from build123d import *

# Parameters (mm, degrees)
F0_R     = 2
F1_DEPTH = 3.2


with BuildPart() as f1:
    # F0 (on Top) → F1 (new body)
    with BuildSketch(Plane.XY):
        with BuildLine():
            ThreePointArc((0, 4), (1.171573, 1.171573), (4, 0))
            Line((4, 0), (76, 0))
            ThreePointArc((76, 0), (78.828427, 1.171573), (80, 4))
            Line((80, 4), (80, 86.6))
            ThreePointArc((80, 86.6), (78.828427, 89.428427), (76, 90.6))
            Line((76, 90.6), (4, 90.6))
            ThreePointArc((4, 90.6), (1.171573, 89.428427), (0, 86.6))
            Line((0, 86.6), (0, 4))
        make_face()
        with Locations((4, 4.8)):
            Circle(F0_R, mode=Mode.SUBTRACT)
        with Locations((4, 20.8)):
            Circle(F0_R, mode=Mode.SUBTRACT)
        with Locations((4, 36.8)):
            Circle(F0_R, mode=Mode.SUBTRACT)
        with Locations((76, 4.8)):
            Circle(F0_R, mode=Mode.SUBTRACT)
        with Locations((76, 20.8)):
            Circle(F0_R, mode=Mode.SUBTRACT)
        with Locations((76, 36.8)):
            Circle(F0_R, mode=Mode.SUBTRACT)
        with Locations((4, 52.8)):
            Circle(F0_R, mode=Mode.SUBTRACT)
        with Locations((4, 68.8)):
            Circle(F0_R, mode=Mode.SUBTRACT)
        with Locations((4, 84.8)):
            Circle(F0_R, mode=Mode.SUBTRACT)
        with Locations((76, 52.8)):
            Circle(F0_R, mode=Mode.SUBTRACT)
        with Locations((76, 68.8)):
            Circle(F0_R, mode=Mode.SUBTRACT)
        with Locations((76, 84.8)):
            Circle(F0_R, mode=Mode.SUBTRACT)
    extrude(amount=F1_DEPTH)


solid = f1.part
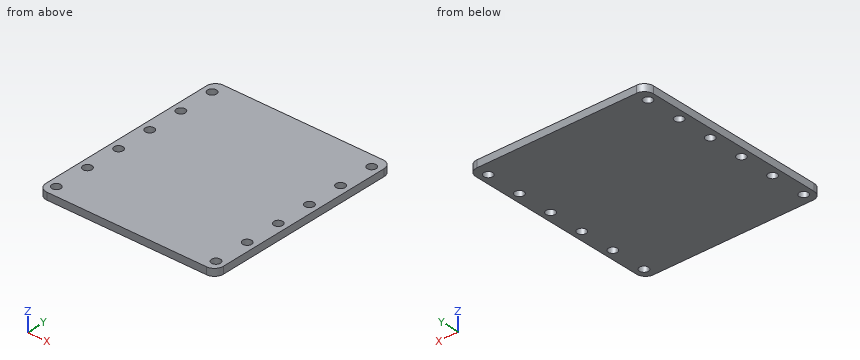
Geometry: final body of the model. Coordinates: model frame, mm. Coordinates: 2 decimals unless noted, no trailing zeros. Order: outer loops, then holes, each group sorted by start corner. A loop starts at its lowest first (then second) coordinate and runs counter-clockwise, first axis right, second up.
(1) Section query B-B (z = 1.7). State how many separate pieces and enclosed holes the cut face has, plus the area to 3 significant figures.
(2) Section query A-A (y = 84.8). Return the cut outline in (x, z).
(3) Material intervals for probe 1 along X at (y, z) = (84.5, 2.6); probe 2 along X at (y, z) = (21.5, 0.7), sorted ascending.
Solution:
1. separate pieces: 1
1. enclosed holes: 12
1. area: 7,080 mm2
2. outline: (0, 0) - (2, 0) - (2, 3.2) - (0, 3.2) - close; (6, 0) - (74, 0) - (74, 3.2) - (6, 3.2) - close; (78, 0) - (80, 0) - (80, 3.2) - (78, 3.2) - close
3. probe 1: x = 0 to 2.02, 5.98 to 74.02, 77.98 to 80
3. probe 2: x = 0 to 2.13, 5.87 to 74.13, 77.87 to 80
